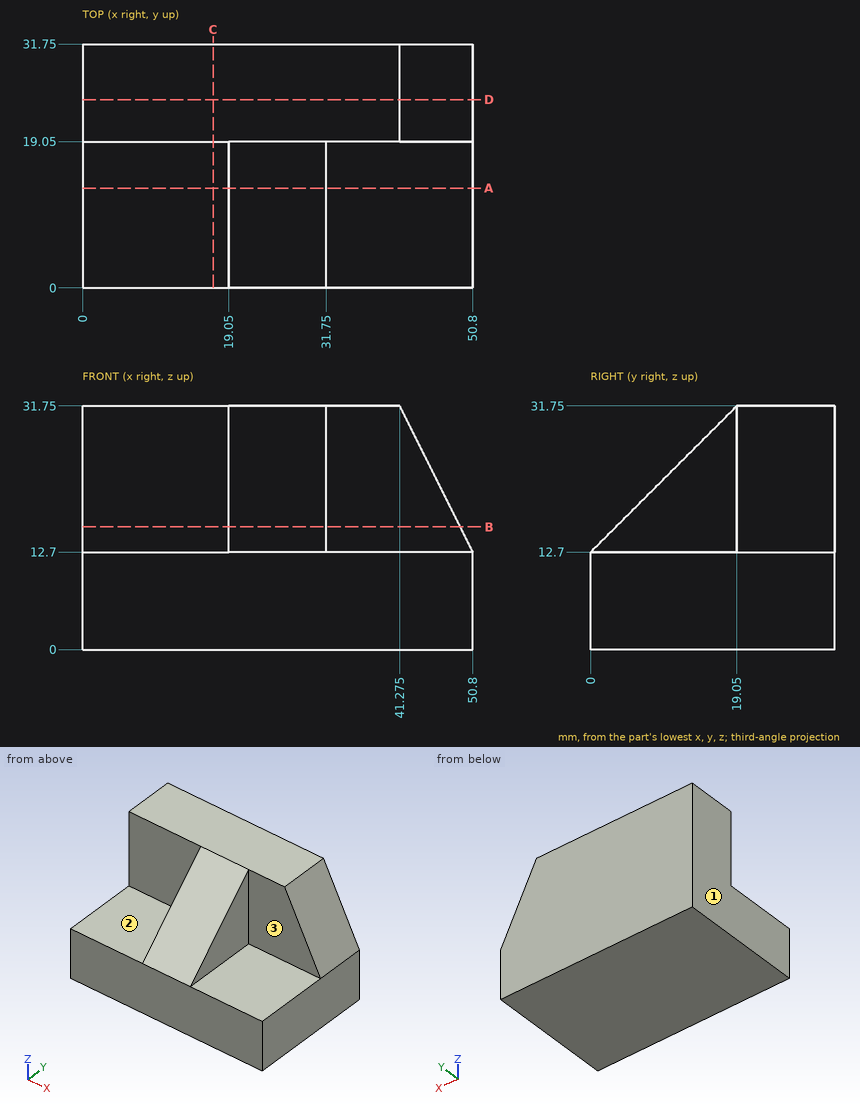
Drawing for the job (mm, zero at the part's lowest x, y, z). A direction names the side the tool comes from. Give positions to 0.01 mm unless a question says otherwise; leave off trailing zeros. Loops run counter-clockwise (first coordinate to the right, second up) from the corner with the lowest first, then second, coordinate; pieces in that order, holes last.
1) Drop flat-ended pins along their axis: P1, Ø15, axis at x = 42.5, z = 20.5, coming from the -Y side; P2, Ø9.5, axis at x = 12, y = 6, coming from the +Z side; P3, Ø9.5, axis at y = 7.5, z = 21.5, coming from the -X side. Give the stop position or say it passes through.
Values follow:
P1: stops at y = 19.05
P2: stops at z = 12.7
P3: stops at x = 19.05
2) Band-saw the part on A-A on y = 13. List the corners of the cut face in (x, z), then the cut area to 3 significant figures.
Values follow:
outline: (0, 0) - (50.8, 0) - (50.8, 12.7) - (31.75, 12.7) - (31.75, 25.7) - (19.05, 25.7) - (19.05, 12.7) - (0, 12.7) - close
area: 810 mm2
3) 3-axis set-ups, long thin cutter, end or side, ignore diameter. For the marked faces 1, 2 and 3: which of +Z, -Z, +X, -X, +Y, -Y reach the whole face in a straight line?
Values follow:
face 1: +Z, -Z, -X, +Y, -Y
face 2: +Z, -X, -Y
face 3: +Z, +X, -Y
4) Band-saw the part on D-D on y = 24.5. List the corners of the cut face in (x, z) (3 decimals), then the cut area to 3 significant figures.
Values follow:
outline: (0, 0) - (50.8, 0) - (50.8, 12.7) - (41.275, 31.75) - (0, 31.75) - close
area: 1,520 mm2
5) Band-saw the part on B-B on z = 16. List the corners of the cut face in (x, y), then the cut area to 3 significant figures.
Values follow:
outline: (0, 19.05) - (19.05, 19.05) - (19.05, 3.3) - (31.75, 3.3) - (31.75, 19.05) - (49.15, 19.05) - (49.15, 31.75) - (0, 31.75) - close
area: 824 mm2
6) Probe line 1 along Y through (x, z) = (15, 14.5); line 2 along Z through (x, y) = (32.5, 10.5). List the from-to ranges inside material, lowest first.
Values follow:
line 1: y = 19.05 to 31.75
line 2: z = 0 to 12.7
7) Band-saw the part on C-C on x = 17. List the corners of the cut face in (y, z).
Values follow:
outline: (0, 0) - (31.75, 0) - (31.75, 31.75) - (19.05, 31.75) - (19.05, 12.7) - (0, 12.7) - close
